Could you check a few things on this model? Use its own coordinates, in mm. A direction names the side the tool comes from. Give positions to 0.01 mm unless a question says otherwise; leave off trailing zeros. Loops run counter-clockwise (first coordinate to the right, second up) from the corner with the lowest first, then second, coordinate; pieces in that order, holes last. Notation, with made-up numbers: (72.5, -13) - (127.5, -13) arc R25 ccw to (127.5, 14) - close; hole circle Ø9 at (50, -37.75). An arc over 180 degrees is marked (long way). Write each question's results on one line, items separated by ' | '. Start each with the question number.
1) I want a section at D-D, the plane z = 18. Write out the boundary of the cut face in (x, y).
2) If I drill on probe 1 along X at (y, z) = (50, 2.9); probe 2 along Y at (x, z) = (50, 7.25), over which ranges is the centre line in solid material (lowest first)? Write a range as [from, to].
3) I want a section at B-B, the plane x = 50. Write out the boundary of the cut face in (y, z), and give its area (3 significant figures).
4) I want a section at A-A, the plane x = 0. Write out the boundary of the cut face in (y, z), and give its area (3 significant figures).
5) On a 3-axis mill with a long thin cutter (end or side, diameter ignored), from which of +Z, -Z, +X, -X, +Y, -Y can I reach the whole of each face in a straight line? I mean faces 4 (the face through (53, 51, 5)), 5 (the face through (-2.222, -10.006, 19.035)), 6 (the face through (47.79, -47.97, 7.54)). Say none if no direction works.
6) I'm going to push flat-ended pins straight in: pin 1 (1.8 mm diameter, centred on y = 2.5, z = 14, fed in from -X); pin 2 (0.7 mm diameter, centred on x = -3, z = 15, fed in from +Y); pin 3 (0.7 mm diameter, centred on x = 3.5, z = 14.5, fed in from +Y). Where does each tip first touch, or does it pass through?
7) If we mould it in two halves opening along X, with no side actions, what happens to faces 1 (the face through (10, 4, 21.5)), 2 (the face through (47.79, 52.03, 7.54)), 3 (the face through (60, -1, 5))? For each: +X half, -X half, draft (parallel to the pull), parting line (faces both ways), or undercut.
from build123d import *

# Parameters (mm, degrees)
F0_W      = 60
F0_H      = 60
F1_DEPTH  = 10
F2_R      = 3
F3_DEPTH  = 25
F4_R      = 4.5
F5_DEPTH  = 5
F6_R      = 13
F7_DEPTH  = 11.5
F8_R      = 4.5
F9_DEPTH  = 25
F10_W     = 8.2
F10_H     = 8.2
F11_DEPTH = 9.2
F12_R     = 10.25
F13_DEPTH = 5


with BuildPart() as f1:
    # F0 (on Top) → F1 (new body)
    with BuildSketch(Plane.XY):
        with Locations((-30, 30)):
            Rectangle(F0_W, F0_H)
        with Locations((-30, -30)):
            Rectangle(F0_W, F0_H)
        with Locations((30, 30)):
            Rectangle(F0_W, F0_H)
        with Locations((30, -30)):
            Rectangle(F0_W, F0_H)
    extrude(amount=F1_DEPTH)

    # F2 (on face) → F3 (cut)
    with BuildSketch(Plane.XY.offset(10)):
        with Locations((-50, 50)):
            Circle(F2_R)
        with Locations((50, 50)):
            Circle(F2_R)
        with Locations((-50, -50)):
            Circle(F2_R)
        with Locations((50, -50)):
            Circle(F2_R)
    extrude(amount=-F3_DEPTH, mode=Mode.SUBTRACT)

    # F4 (on face) → F5 (cut)
    with BuildSketch(Plane(origin=(0, 0, 0), x_dir=(1, 0, 0), z_dir=(0, 0, -1))):
        with Locations((-50, 50)):
            Circle(F4_R)
        with Locations((50, 50)):
            Circle(F4_R)
        with Locations((-50, -50)):
            Circle(F4_R)
        with Locations((50, -50)):
            Circle(F4_R)
    extrude(amount=-F5_DEPTH, mode=Mode.SUBTRACT)

    # F6 (on face) → F7 (join)
    with BuildSketch(Plane.XY.offset(10)):
        Circle(F6_R)
    extrude(amount=F7_DEPTH)

    # F8 (on face) → F9 (cut)
    with BuildSketch(Plane.XY.offset(21.5)):
        Circle(F8_R)
    extrude(amount=-F9_DEPTH, mode=Mode.SUBTRACT)

    # F10 (on face) → F11 (cut)
    with BuildSketch(Plane.XY.offset(21.5)):
        Rectangle(F10_W, F10_H)
    extrude(amount=-F11_DEPTH, mode=Mode.SUBTRACT)

    # F12 (on face) → F13 (cut)
    with BuildSketch(Plane.XY.offset(21.5)):
        Circle(F12_R)
    extrude(amount=-F13_DEPTH, mode=Mode.SUBTRACT)


solid = f1.part
Answers:
1) outline: circle Ø26 at (0, 0); hole circle Ø20.5 at (0, 0)
2) probe 1: x = [-60, -54.5], [-45.5, 45.5], [54.5, 60] | probe 2: y = [-60, -53], [-47, 47], [53, 60]
3) outline: (-60, 0) - (-54.5, 0) - (-54.5, 5) - (-53, 5) - (-53, 10) - (-60, 10) - close; (-47, 5) - (-45.5, 5) - (-45.5, 0) - (45.5, 0) - (45.5, 5) - (47, 5) - (47, 10) - (-47, 10) - close; (53, 5) - (54.5, 5) - (54.5, 0) - (60, 0) - (60, 10) - (53, 10) - close | area: 1,050 mm2
4) outline: (-60, 0) - (-4.5, 0) - (-4.5, 16.5) - (-10.25, 16.5) - (-10.25, 21.5) - (-13, 21.5) - (-13, 10) - (-60, 10) - close; (4.5, 0) - (60, 0) - (60, 10) - (13, 10) - (13, 21.5) - (10.25, 21.5) - (10.25, 16.5) - (4.5, 16.5) - close | area: 1,250 mm2
5) face 4: -Z | face 5: +Z | face 6: +Z, -Z
6) pin 1: stops at x = -12.9 | pin 2: stops at y = 12.73 | pin 3: stops at y = 12.61
7) face 1: draft | face 2: undercut | face 3: +X half
